Can you work these out from the model? Positions are in its coordinate system, mm. A direction names the side the tool comes from. Give positions to 0.01 mm unless a question says otherwise; leave off trailing zeros. Write each loop counter-clockwise with the first axis right and the second up, starting at its lowest first coordinate (ties: lowest second). Pieces come first, ordered by that corner, then holes.
1. On a 3-axis mill with a long thin cutter (end or side, diameter ignored), from which of +Z, -Z, +X, -X, +Y, -Y can I reach the whole of each face in a straight line? I mean faces 5 (the cylindrical face through (-2.728, 20.777, 3.28)), 6 (the flat face through (-15, -10, 0)), 7 (the cylindrical face through (-18, 10.095, 0.845)). Say none if no direction works.
2. Suppose I cut it at C-C (y = -20). Please give me the cut outline in (x, z).
3. Suppose I cut it at D-D (z = 3.85). Please give me the cut outline in (x, y) (1 decimal), and give its area (3 significant figures).
4. Thinking about a two-plate mould opening in X: for faces 1 (the flat face through (1.7, -21.1, 4.89)), 2 (the cylindrical face through (-0.07, 17.218, 0.845)), 3 (the cylindrical face through (14.946, -8.548, 0.845)), 4 (the cylindrical face through (0.07, 28.375, 0.845)), which applies, pulls with the +X half, pulls with the -X half, needs draft (parallel to the pull), parting line crosses it, or undercut?
5. I'm going to push a flat-ended pin straight in: pin 1 (2 mm diameter, centred on y = 9, z = 1, fed in from +X). Where does the tip first touch, or does it pass through?
6. If I drill on probe 1 along Y at (x, z) = (0, 2.6) (1 decimal); probe 2 along X at (y, z) = (19, 0.2); probe 3 along X at (y, z) = (-10.5, 2.35), over which ranges is the centre line in solid material (lowest first)?
```python
from build123d import *

# Parameters (mm, degrees)
F1_DEPTH = 1.7145
F2_R     = 23.8125
F2_R_2   = 20.955
F3_DEPTH = 3.175


with BuildPart() as f1:
    # F0 (on Top) → F1 (new body)
    with BuildSketch(Plane.XY):
        with BuildLine():
            ThreePointArc((-3.175, 25.2007812379), (-16.8005208253, -19.05), (25.4, 0))
            ThreePointArc((25.4, 0), (19.05, 16.8005208253), (3.175, 25.2007812379))
            ThreePointArc((3.175, 25.2007812379), (0, 25.4), (-3.175, 25.2007812379))
        make_face()
        with BuildLine():
            ThreePointArc((3.175, 20.3918067186), (15.6753065161, 13.4235305294), (20.6375, 0))
            ThreePointArc((20.6375, 0), (20.2869789198, -3.7874651889), (19.2473226474, -7.4462727023))
            ThreePointArc((19.2473226474, -7.4462727023), (17.8725992706, -10.31875), (16.0723226474, -12.9455340163))
            ThreePointArc((16.0723226474, -12.9455340163), (0, -20.6375), (-16.0723226474, -12.9455340163))
            ThreePointArc((-16.0723226474, -12.9455340163), (-17.8725992706, -10.31875), (-19.2473226474, -7.4462727023))
            ThreePointArc((-19.2473226474, -7.4462727023), (-17.8725992706, 10.31875), (-3.175, 20.3918067186))
            ThreePointArc((-3.175, 20.3918067186), (0, 20.6375), (3.175, 20.3918067186))
        make_face(mode=Mode.SUBTRACT)
        with BuildLine():
            ThreePointArc((-3.175, 20.3918067186), (0, 17.2168067186), (3.175, 20.3918067186))
            ThreePointArc((3.175, 20.3918067186), (0, 20.6375), (-3.175, 20.3918067186))
        make_face()
        with BuildLine():
            ThreePointArc((-16.0723226474, -12.9455340163), (-14.9101919904, -8.6084033593), (-19.2473226474, -7.4462727023))
            ThreePointArc((-19.2473226474, -7.4462727023), (-17.8725992706, -10.31875), (-16.0723226474, -12.9455340163))
        make_face()
        with BuildLine():
            ThreePointArc((16.0723226474, -12.9455340163), (17.8725992706, -10.31875), (19.2473226474, -7.4462727023))
            ThreePointArc((19.2473226474, -7.4462727023), (14.9101919904, -8.6084033593), (16.0723226474, -12.9455340163))
        make_face()
        with BuildLine():
            ThreePointArc((-3.175, 25.2007812379), (0, 25.4), (3.175, 25.2007812379))
            ThreePointArc((3.175, 25.2007812379), (0, 28.3757812379), (-3.175, 25.2007812379))
        make_face()
    extrude(amount=F1_DEPTH)

    # F2 (on face) → F3 (join)
    with BuildSketch(Plane.XY.offset(1.7145)):
        Circle(F2_R)
        Circle(F2_R_2, mode=Mode.SUBTRACT)
    extrude(amount=F3_DEPTH)


solid = f1.part
```
Checks:
1. face 5: +Z
1. face 6: -Z, +X, -X, +Y, -Y
1. face 7: +Z, -Z
2. outline: (-15.66, 0) - (-5.09, 0) - (-5.09, 1.71) - (-6.25, 1.71) - (-6.25, 4.89) - (-12.92, 4.89) - (-12.92, 1.71) - (-15.66, 1.71) - close; (5.09, 0) - (15.66, 0) - (15.66, 1.71) - (12.92, 1.71) - (12.92, 4.89) - (6.25, 4.89) - (6.25, 1.71) - (5.09, 1.71) - close
3. outline: circle Ø47.6 at (0, 0); hole circle Ø41.9 at (0, 0)
3. area: 402 mm2
4. face 1: needs draft
4. face 2: undercut
4. face 3: undercut
4. face 4: parting line crosses it
5. pin 1: stops at x = 24.11
6. probe 1: y = -23.8 to -21, 21 to 23.8
6. probe 2: x = -16.86 to -8.06, -2.85 to 2.85, 8.06 to 16.86
6. probe 3: x = -21.37 to -18.13, 18.13 to 21.37
